Autodesk Inventor part; units mm, degrees
ref_plane "YZ Plane" through (0, 0, 0) normal (1, 0, 0) x (0, 1, 0)
ref_plane "XZ Plane" through (0, 0, 0) normal (0, 1, 0) x (-1, 0, 0)
ref_plane "XY Plane" through (0, 0, 0) normal (0, 0, 1) x (1, 0, 0)
sketch "Sketch1" plane through (0, 0, 0) normal (0, 1, 0) x (-1, 0, 0)
  line L0 (31.1634, 169.1828) -> (-118.8366, 169.1828)
  line L1 (-118.8366, 169.1828) -> (-118.8366, -80.8172)
  line L2 (-118.8366, -80.8172) -> (31.1634, -80.8172)
  line L3 (31.1634, -80.8172) -> (31.1634, 169.1828)
  point P0 (0, 0)
  dimension "d0" = 250
  dimension "d1" = 150
extrude "Extrusion1" add sketch "Sketch1" along normal blind 4
fillet "Fillet1" [suppressed]
sketch "Sketch2" plane through (0, 4, 0) normal (0, 1, 0) x (1, 0, 0)
  line L0 (-31.1634, 80.8172) -> (-31.1634, -169.1828)
  line L1 (-31.1634, -169.1828) -> (118.8366, -169.1828)
  line L2 (118.8366, -169.1828) -> (118.8366, 80.8172)
  line L3 (118.8366, 80.8172) -> (-31.1634, 80.8172)
  arc A0 (-21.1634, 76.8172) -> (-27.1634, 70.8172) centre (-21.1634, 70.8172) ccw
  arc A1 (114.8366, 70.8172) -> (108.8366, 76.8172) centre (108.8366, 70.8172) ccw
  arc A2 (108.8366, -165.1828) -> (114.8366, -159.1828) centre (108.8366, -159.1828) ccw
  arc A3 (-27.1634, -159.1828) -> (-21.1634, -165.1828) centre (-21.1634, -159.1828) ccw
  line L4 (108.8366, -165.1828) -> (98.8366, -165.1828)
  line L5 (-11.1634, -165.1828) -> (-21.1634, -165.1828)
  line L6 (-27.1634, -159.1828) -> (-27.1634, -149.1828)
  line L7 (-27.1634, 60.8172) -> (-27.1634, 70.8172)
  line L8 (-21.1634, 76.8172) -> (-11.1634, 76.8172)
  line L9 (98.8366, 76.8172) -> (108.8366, 76.8172)
  line L10 (114.8366, 70.8172) -> (114.8366, 60.8172)
  line L11 (114.8366, -149.1828) -> (114.8366, -159.1828)
  line L12 (-11.1634, -169.1828) -> (-11.1634, -165.1828)
  line L13 (-11.1634, 76.8172) -> (-11.1634, 80.8172)
  line L14 (-31.1634, 60.8172) -> (-27.1634, 60.8172)
  line L15 (114.8366, 60.8172) -> (118.8366, 60.8172)
  line L16 (98.8366, -169.1828) -> (98.8366, -165.1828)
  line L17 (98.8366, 76.8172) -> (98.8366, 80.8172)
  line L18 (-31.1634, -149.1828) -> (-27.1634, -149.1828)
  line L19 (114.8366, -149.1828) -> (118.8366, -149.1828)
  point P0 (0, 0)
  point P1 (114.8366, -154.1828)
  dimension "d12" = 4
  dimension "d13" = 20
  dimension "d14" = 4
extrude "Extrusion2" [suppressed]
sketch "Sketch3" plane through (0, 4, 0) normal (0, 1, 0) x (1, 0, 0)
  line L0 (-29.1634, -129.1828) -> (-27.1634, -129.1828)
  line L1 (-27.1634, -129.1828) -> (-27.1634, -109.1828)
  line L2 (-27.1634, -109.1828) -> (-29.1634, -109.1828)
  line L3 (-29.1634, -109.1828) -> (-29.1634, -129.1828)
  line L4 (-31.1634, 80.8172) -> (-31.1634, -169.1828)
  line L5 (-29.1634, -71.6828) -> (-29.1634, -91.6828)
  line L6 (-29.1634, -91.6828) -> (-27.1634, -91.6828)
  line L7 (-27.1634, -91.6828) -> (-27.1634, -71.6828)
  line L8 (-27.1634, -71.6828) -> (-29.1634, -71.6828)
  line L9 (-29.1634, -34.1828) -> (-29.1634, -54.1828)
  line L10 (-29.1634, -54.1828) -> (-27.1634, -54.1828)
  line L11 (-27.1634, -54.1828) -> (-27.1634, -34.1828)
  line L12 (-27.1634, -34.1828) -> (-29.1634, -34.1828)
  line L13 (-29.1634, 3.3172) -> (-29.1634, -16.6828)
  line L14 (-29.1634, -16.6828) -> (-27.1634, -16.6828)
  line L15 (-27.1634, -16.6828) -> (-27.1634, 3.3172)
  line L16 (-27.1634, 3.3172) -> (-29.1634, 3.3172)
  line L17 (-29.1634, 40.8172) -> (-29.1634, 20.8172)
  line L18 (-29.1634, 20.8172) -> (-27.1634, 20.8172)
  line L19 (-27.1634, 20.8172) -> (-27.1634, 40.8172)
  line L20 (-27.1634, 40.8172) -> (-29.1634, 40.8172)
  line L21 (-31.1634, -169.1828) -> (118.8366, -169.1828)
  line L22 (114.8366, -129.1828) -> (116.8366, -129.1828)
  line L23 (116.8366, -129.1828) -> (116.8366, -109.1828)
  line L24 (116.8366, -109.1828) -> (114.8366, -109.1828)
  line L25 (114.8366, -109.1828) -> (114.8366, -129.1828)
  line L26 (114.8366, -91.6828) -> (116.8366, -91.6828)
  line L27 (114.8366, -71.6828) -> (114.8366, -91.6828)
  line L28 (116.8366, -71.6828) -> (114.8366, -71.6828)
  line L29 (114.8366, -54.1828) -> (116.8366, -54.1828)
  line L30 (116.8366, -34.1828) -> (114.8366, -34.1828)
  line L31 (114.8366, -34.1828) -> (114.8366, -54.1828)
  line L32 (116.8366, -54.1828) -> (116.8366, -34.1828)
  line L33 (116.8366, -91.6828) -> (116.8366, -71.6828)
  line L34 (114.8366, -16.6828) -> (116.8366, -16.6828)
  line L35 (116.8366, -16.6828) -> (116.8366, 3.3172)
  line L36 (114.8366, 3.3172) -> (114.8366, -16.6828)
  line L37 (116.8366, 3.3172) -> (114.8366, 3.3172)
  line L38 (114.8366, 20.8172) -> (116.8366, 20.8172)
  line L39 (114.8366, 40.8172) -> (114.8366, 20.8172)
  line L40 (116.8366, 40.8172) -> (114.8366, 40.8172)
  line L41 (116.8366, 20.8172) -> (116.8366, 40.8172)
  line L42 (-1.1634, -167.1828) -> (18.8366, -167.1828)
  line L43 (18.8366, -167.1828) -> (18.8366, -165.1828)
  line L44 (18.8366, -165.1828) -> (-1.1634, -165.1828)
  line L45 (-1.1634, -165.1828) -> (-1.1634, -167.1828)
  line L46 (53.8366, -167.1828) -> (53.8366, -165.1828)
  line L47 (53.8366, -165.1828) -> (33.8366, -165.1828)
  line L48 (33.8366, -167.1828) -> (53.8366, -167.1828)
  line L49 (33.8366, -165.1828) -> (33.8366, -167.1828)
  line L50 (88.8366, -167.1828) -> (88.8366, -165.1828)
  line L51 (88.8366, -165.1828) -> (68.8366, -165.1828)
  line L52 (68.8366, -167.1828) -> (88.8366, -167.1828)
  line L53 (68.8366, -165.1828) -> (68.8366, -167.1828)
  line L54 (18.8366, 76.8172) -> (18.8366, 78.8172)
  line L55 (18.8366, 78.8172) -> (-1.1634, 78.8172)
  line L56 (-1.1634, 76.8172) -> (18.8366, 76.8172)
  line L57 (-1.1634, 78.8172) -> (-1.1634, 76.8172)
  line L58 (53.8366, 76.8172) -> (53.8366, 78.8172)
  line L59 (53.8366, 78.8172) -> (33.8366, 78.8172)
  line L60 (33.8366, 76.8172) -> (53.8366, 76.8172)
  line L61 (33.8366, 78.8172) -> (33.8366, 76.8172)
  line L62 (88.8366, 76.8172) -> (88.8366, 78.8172)
  line L63 (88.8366, 78.8172) -> (68.8366, 78.8172)
  line L64 (68.8366, 76.8172) -> (88.8366, 76.8172)
  line L65 (68.8366, 78.8172) -> (68.8366, 76.8172)
  point P0 (0, 0)
  dimension "d15" = 2
  dimension "d16" = 20
  dimension "d17" = 2
  dimension "d21" = 37.5
  dimension "d28" = 144
  dimension "d33" = 20
  dimension "d34" = 2
  dimension "d35" = 2
  dimension "d39" = 35
  dimension "d42" = 244
extrude "Extrusion3" cut sketch "Sketch3" against normal through all
sketch "Sketch4" plane through (0, 4, 0) normal (0, 1, 0) x (1, 0, 0)
  circle A0 centre (98.8366, -134.1828) radius 9.6
  line L0 (118.8366, -169.1828) -> (118.8366, 80.8172)
  line L1 (-31.1634, -169.1828) -> (118.8366, -169.1828)
  line L2 (91.7366, -92.6828) -> (105.9366, -92.6828)
  line L3 (105.9366, -92.6828) -> (105.9366, -115.6828)
  line L4 (105.9366, -115.6828) -> (91.7366, -115.6828)
  line L5 (91.7366, -115.6828) -> (91.7366, -92.6828)
  circle A1 centre (98.8366, -19.1828) radius 8.1
  line L6 (-31.1634, 80.8172) -> (-31.1634, -169.1828)
  circle A2 centre (98.8366, 10.8172) radius 4.1
  line L7 (90.9866, -150.9828) -> (106.6866, -150.9828)
  line L8 (106.6866, -150.9828) -> (106.6866, -159.1828)
  line L9 (106.6866, -159.1828) -> (90.9866, -159.1828)
  line L10 (90.9866, -159.1828) -> (90.9866, -150.9828)
  circle A3 centre (98.8366, -117.6828) radius 1.5
  circle A4 centre (98.8366, -90.6828) radius 1.5
  circle A5 centre (109.0866, -155.0828) radius 1.5
  circle A6 centre (88.5866, -155.0828) radius 1.5
  point P0 (0, 0)
  point P1 (105.9366, -104.1828)
  point P2 (98.8366, -115.6828)
  point P3 (91.7366, -104.1828)
  point P4 (98.8366, -150.9828)
  dimension "d47" = 19.2
  dimension "d50" = 20
  dimension "d51" = 35
  dimension "d52" = 14.2
  dimension "d53" = 23
  dimension "d54" = 30
  dimension "d56" = 0
  dimension "d57" = 16.2
  dimension "d59" = 130
  dimension "d60" = 150
  dimension "d61" = 8.2
  dimension "d62" = 30
  dimension "d73" = 15.7
  dimension "d74" = 8.2
  dimension "d75" = 0
  dimension "d76" = 10
  dimension "d89" = 3
  dimension "d90" = 3
  dimension "d91" = 27
  dimension "d92" = 13.5
  dimension "d93" = 3
  dimension "d94" = 3
  dimension "d95" = 20.5
  dimension "d96" = 10.25
extrude "Extrusion4" cut sketch "Sketch4" against normal blind 10
sketch "Sketch5" plane through (0, 4, 0) normal (0, 1, 0) x (1, 0, 0)
  circle A0 centre (98.8366, -59.1828) radius 5
  circle A1 centre (98.8366, -19.1828) radius 8.1
  point P0 (0, 0)
  dimension "d63" = 10
  dimension "d77" = 40
extrude "Extrusion5" add sketch "Sketch5" along normal blind 8 contours A0
sketch "Sketch6" plane through (98.8366, 12, 59.1828) normal (0, 1, 0) x (1, 0, 0)
  circle A0 centre (0, 0) radius 5
  point P0 (-98.8366, 59.1828)
hole "Hole1" at (98.8366, 12, 59.1828) direction (0, -1, 0) diameter 4 depth 6
sketch "Sketch7" plane through (0, 4, 0) normal (0, 1, 0) x (1, 0, 0)
  circle A0 centre (-27.6634, 77.3172) radius 1.5
  line L0 (118.8366, 80.8172) -> (-31.1634, 80.8172)
  line L1 (-31.1634, 80.8172) -> (-31.1634, -169.1828)
  point P0 (0, 0)
  dimension "d78" = 3
  dimension "d79" = 3.5
  dimension "d80" = 3.5
extrude "Extrusion6" cut sketch "Sketch7" against normal blind 10
pattern_linear "Rectangular Pattern1" count 2 spacing 243 along (0, 0, 1) count 2 spacing 143 along (1, 0, 0) of "Extrusion6"
properties part number "Enclosure_6"
CAD build for the part. Positions are in the model's coordinates, mm. Give positions to 0.01 mm unless a question says otherwise; leave off trailing zeros. Order: outer loops, then holes, each group sorted by start corner. A loop starts at its lowest first (then second) coordinate and runs counter-clockwise, first axis right, second up. Notation, with made-up numbers: M -38.75,-40 L 12.25,-40 A34 ccw 12.25,-2 Z; hole C -25.75,43.25 d6. An arc over 180 degrees is marked long. Put each result on its own line as item: value. Start each with the question number.
(1) Saw through at A-A, the plane z = 102. Write the cut outline in (x, y).
(2) Saw through at D-D, the plane x = 58. Write the cut outline in (y, z).
(3) Mould opens along X. For faces 1 (the flat face through (45, 0, 46)), 2 (the cylindrical face through (95.6, 2, -8.3)), 3 (the cylindrical face through (107.993, 2.028, 131.299)), 4 (the cylindrical face through (93.84, 7.94, 59.4)) say: +X half, -X half, draft (parallel to the pull), parting line (faces both ways), or undercut.
(4) Saw through at B-B, the plane x = 38.5. Write the cut outline in (y, z).
(5) Saw through at C-C, the plane z = -28. Write the cut outline in (x, y).
(6) Flat gauge pins, fed straight in: pin 1 Ø5 at (y, z) = (8, 6) entering from +X; pin 2 Ø6 at (x, z) = (32, -17.5) entering from -Y; pin 3 Ø1.5 at (x, y) = (95.5, 5.5) entering from -Z. Where does each tip first touch, or does it go through?
(7) Drill centre lines: line 1 along Z through (x, y) = (38, 3.25); line 2 along X through (y, z) = (2.25, -26); line 3 along Y through (x, z) = (88.5, 143). Where is each one in solid material? Low to high.
Check result:
1. outline: M -31.16,0 L 91.74,0 L 91.74,4 L -31.16,4 Z; M 105.94,0 L 118.84,0 L 118.84,4 L 105.94,4 Z
2. outline: M 0,-80.82 L 4,-80.82 L 4,169.18 L 0,169.18 Z
3. face 1: draft
3. face 2: undercut
3. face 3: undercut
3. face 4: parting line
4. outline: M 0,-80.82 L 4,-80.82 L 4,-78.82 L 0,-78.82 Z; M 0,-76.82 L 4,-76.82 L 4,165.18 L 0,165.18 Z; M 0,167.18 L 4,167.18 L 4,169.18 L 0,169.18 Z
5. outline: M -31.16,0 L -29.16,0 L -29.16,4 L -31.16,4 Z; M -27.16,0 L 114.84,0 L 114.84,4 L -27.16,4 Z; M 116.84,0 L 118.84,0 L 118.84,4 L 116.84,4 Z
6. pin 1: passes through
6. pin 2: stops at y = 0
6. pin 3: stops at z = 54.9
7. line 1: z = -80.82 to -78.82, -76.82 to 165.18, 167.18 to 169.18
7. line 2: x = -31.16 to -29.16, -27.16 to 114.84, 116.84 to 118.84
7. line 3: y = 0 to 4
